Geometry check sheet. Reference: the model listing, model coordinates, mm. Face numbers are marked on the shaded views. A direction names the side the tool comes from. Give positions to 0.01 mm unless a question says otherwise; leave off trailing zeros. Loops run counter-clockwise (first coordinate to the right, second up) from the corner with the lowest first, then second, coordinate; pieces in that order, holes last. Notation, with made-up numbers: (64.25, 78) -> (91.25, 78) arc R20 ccw to (91.25, 103) -> close; hole circle Ø3 at (42.5, 32). An arc over 180 degrees is marked (long way). Write item = value, one per line. Start each with the question number.
```python
from build123d import *

# Parameters (mm, degrees)
F0_W     = 304.8
F0_H     = 304.8
F1_DEPTH = 38.1
F2_W     = 266.7
F2_H     = 266.7
F3_DEPTH = 50.8


with BuildPart() as f1:
    # F0 (on Top) → F1 (new body, symmetric)
    with BuildSketch(Plane.XY):
        Rectangle(F0_W, F0_H)
    extrude(amount=F1_DEPTH, both=True)

    # F2 (on face) → F3 (cut)
    with BuildSketch(Plane.XY.offset(38.1)):
        Rectangle(F2_W, F2_H)
    extrude(amount=-F3_DEPTH, mode=Mode.SUBTRACT)


solid = f1.part
```
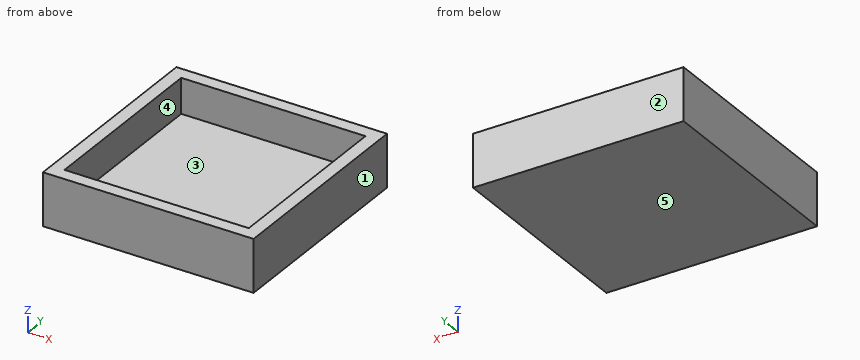
1) Thickness scan on line 1 (Y direction, x = -85.5, z = 9.5); line 2 (Z direction, x = 90, y = -123.5). Record the ranges inside material, lowest first.
2) Tool access check on the marked faces 4 and 5. Record the directions out of +Z, -Z, +X, -X, +Y, -Y that give a thin tool (end or side, any length) a straight path to the whole face; none if there is none.
3) Section check B-B (y = -52.5). Enter the section's corners in (x, z), plus the area to 3 significant figures.
4) Section check A-A (z = 8.5). Enter the section's corners in (x, y).
5) Draft check along X on the marked faces 1, 2 and 3. Enter one of: released by +X, released by -X, zero draft, split by the parting line, or undercut.
Check result:
q1.line_1 = -152.4 to -133.35, 133.35 to 152.4
q1.line_2 = -38.1 to -12.7
q2.face_4 = +Z
q2.face_5 = -Z, +X, -X, +Y, -Y
q3.outline = (-152.4, -38.1) -> (152.4, -38.1) -> (152.4, 38.1) -> (133.35, 38.1) -> (133.35, -12.7) -> (-133.35, -12.7) -> (-133.35, 38.1) -> (-152.4, 38.1) -> close
q3.area = 9,680 mm2
q4.outline = (-152.4, -152.4) -> (152.4, -152.4) -> (152.4, 152.4) -> (-152.4, 152.4) -> close; hole (-133.35, -133.35) -> (133.35, -133.35) -> (133.35, 133.35) -> (-133.35, 133.35) -> close
q5.face_1 = released by +X
q5.face_2 = zero draft
q5.face_3 = undercut
